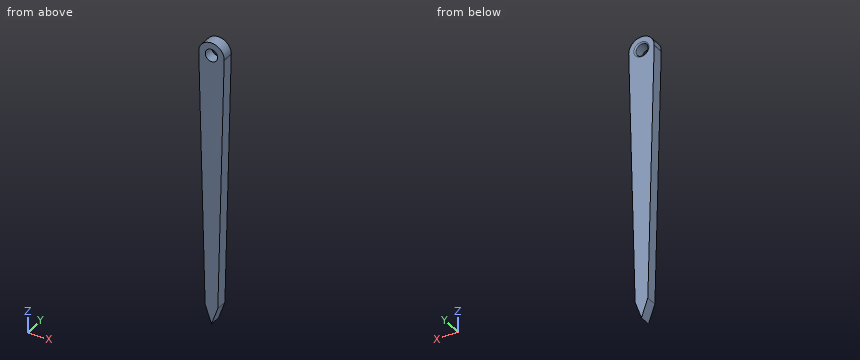
```python
from build123d import *

# Parameters (mm, degrees)
SKICA1_R                 = 1.75
P_IDAT_VYSUNUT_M1_DEPTH  = 3.5
SKICA2_R                 = 1.95
ODEBRAT_VYSUNUT_M1_DEPTH = 100
ZAOBLIT1_R               = 0.4


with BuildPart() as part:
    # Skica1 → Přidat vysunutím1 (new body)
    # profile 1 of 2: a face of its own
    with BuildSketch(Plane(origin=(0, 0, 0), x_dir=(1, 0, 0), z_dir=(0, 1, 0))):
        with BuildLine():
            Line((-2, 80), (-3.995003123, 0.199875078))
            ThreePointArc((-3.995003123, 0.199875078), (0, 4), (3.995003123, 0.199875078))
            Line((3.995003123, 0.199875078), (2, 80))
            Line((2, 80), (0, 85.656854249))
            Line((0, 85.656854249), (-2, 80))
        make_face()
    # profile 2 of 2: a face of its own
    with BuildSketch(Plane(origin=(0, 0, 0), x_dir=(1, 0, 0), z_dir=(0, 1, 0))):
        with BuildLine():
            Line((-3.995003123, 0.199875078), (-4, 0))
            ThreePointArc((-4, 0), (0, -4), (4, 0))
            Line((4, 0), (3.995003123, 0.199875078))
            ThreePointArc((3.995003123, 0.199875078), (0, 4), (-3.995003123, 0.199875078))
        make_face()
        with Locations(Location((0, 0, 0), (0, 0, 270))):
            Circle(SKICA1_R, mode=Mode.SUBTRACT)
    extrude(amount=P_IDAT_VYSUNUT_M1_DEPTH)

    # Skica2 → Odebrat vysunutím1 (cut)
    with BuildSketch(Plane(origin=(0, 3.5, 0), x_dir=(1, 0, 0), z_dir=(0, 1, 0))):
        with Locations(Location((0, 0, 0), (0, 0, 270))):
            Circle(SKICA2_R)
    extrude(amount=-ODEBRAT_VYSUNUT_M1_DEPTH, mode=Mode.SUBTRACT)

    # Zaoblit1
    zaoblit1_edges = [part.edges().sort_by_distance(p)[0] for p in [
        (0, 3.5, -1.95),
    ]]
    fillet(zaoblit1_edges, radius=ZAOBLIT1_R)


solid = part.part
```
Here's how the part is built. I have some questions about the finished solid (model axes, mm). Coordinates: 2 decimals unless noted, no trailing zeros. Loops run counter-clockwise (first coordinate to the right, second up) from the corner with the lowest first, then second, coordinate; pieces in that order, holes last. Notation, with made-up numbers: (-38.5, 63.5) - (5.5, 63.5) arc R19 ccw to (5.5, 67.5) - close; hole circle Ø3 at (58.25, 83). An arc over 180 degrees is marked (long way). Return JSON: item names as keys, results as strings. Group by question number.
Item 1: Will these pins go through, and if not, where does the flat tip stop? P1, Ø1, axis at x = -1.5, y = 1, coming from the +Z side; P2, Ø1.5, axis at y = 2.5, z = -33, coming from the -X side; P3, Ø1, axis at x = 2, y = 0.5, coming from the +Z side.
Item 2: I need wall thicknesses on line 1 (X direction, y = 2.65, z = -7) (3 decimals); line 2 (X direction, y = 3.25, z = -55.5). Which ranges of each line are inside material? Lowest first, please. Write a range as from..to.
Item 3: If we section it at B-B on z = -77: Write out the boundary of the cut face in (x, y) (3 decimals), and give its area (3 significant figures).
Item 4: If we section it at A-A on y = 0.8: Write out the boundary of the cut face in (x, z) (3 decimals).
Item 5: If we section it at C-C on z = -5: Write out the boundary of the cut face in (x, y) (3 decimals).
Calculated:
{
 "1": {"P1": "stops at z = 3.87", "P2": "stops at x = -3.19", "P3": "stops at z = 3.71"},
 "2": {"line 1": "x = -3.825..3.825", "line 2": "x = -2.61..2.61"},
 "3": {"outline": "(-2.075, 0) - (2.075, 0) - (2.075, 3.5) - (-2.075, 3.5) - close", "area": "14.5 mm^2"},
 "4": {"outline": "(-4, 0) - (-2, -80) - (0, -85.657) - (2, -80) - (4, 0) arc R4 ccw to start; hole circle Ø3.9 at (0, 0)"},
 "5": {"outline": "(-3.875, 0) - (3.875, 0) - (3.875, 3.5) - (-3.875, 3.5) - close"}
}
